For this review, take the finished solid that the model builds, in its own axes (mm). Face numbers are marked on the shaded views. Coordinates: 2 decimals unless noted, no trailing zeros. Loops run counter-clockwise (first coordinate to the right, second up) from the corner with the lowest first, then second, coordinate; pieces in that order, holes last. Notation, with made-up numbers: M 68.5,-33 L 100.5,-33 A26 cw 100.5,3 Z; hole C -7.75,46 d1. An arc over 180 degrees is marked long. Answer as a JSON object with one key per item and string values. Group by question number.
Item 1: Add section C-C (z = -20). State the section outline as (x, y) points.
Item 2: Add section D-D (x = 64.5). State the section outline as (y, z) points.
Item 3: Insertion check: pin 1 (1 mm diameter, centred on x = 36, z = -32.5, fed in from -Y). The pin has a flat end and moves straight along its axis. Give the tip position at first contact, or say it passes through.
Item 4: Add section A-A (y = -3.95). State the section outline as (x, z) points, then the cut area to 3 significant figures.
Item 5: Mouldability with a two-part tool opening along X and no side actions: class the marked faces 1 and 2 as +X half, -X half, draft (parallel to the pull), parting line (faces both ways), or undercut.
Item 6: Add section B-B (x = 26). State the section outline as (y, z) points.
Item 7: Wall thickness on L1, parallel to Z at x = 60.5, y = -2.7; L2, parallel to X at y = -3.3, z = -19; L3, parallel to X at y = -3.65, z = -7.5: over which ranges is each line inside the solid? List them lowest first. Write a range as from..to.
from build123d import *

# Parameters (mm, degrees)
F0_W     = 76.2
F0_H     = 38.1
F1_DEPTH = 5.08
F2_W     = 72.268962
F2_H     = 32.798988
F3_DEPTH = 2.54
F4_R     = 10.16
F5_DEPTH = 2.54


with BuildPart() as f1:
    # F0 (on Front) → F1 (new body)
    with BuildSketch(Plane.XZ):
        with Locations((38.1, -19.05)):
            Rectangle(F0_W, F0_H)
    extrude(amount=F1_DEPTH)

    # F2 (on face) → F3 (cut)
    with BuildSketch(Plane.XZ.offset(5.08)):
        with Locations((37.983545, -18.917193)):
            Rectangle(F2_W, F2_H)
    extrude(amount=-F3_DEPTH, mode=Mode.SUBTRACT)

    # F4 (on face) → F5 (join)
    with BuildSketch(Plane.XZ.offset(2.54)):
        with Locations((13.917368, -18.489809)):
            Circle(F4_R)
        with Locations((36.991507, -18.844597)):
            Circle(F4_R)
        with Locations((60.718681, -18.846158)):
            Circle(F4_R)
    extrude(amount=F5_DEPTH)


solid = f1.part
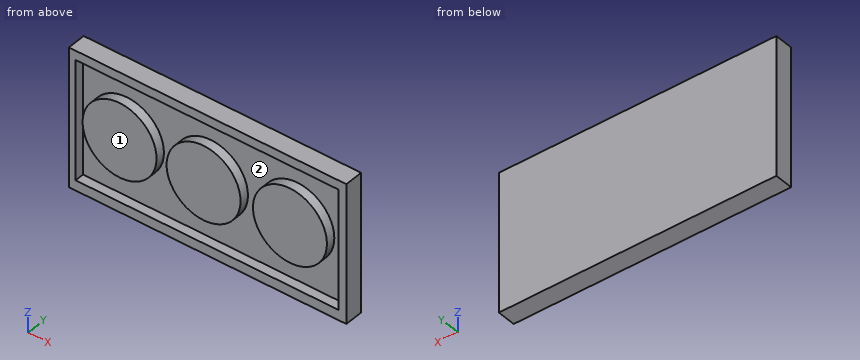
From the geometry:
{
 "1": {"outline": "M 0,-5.08 L 1.85,-5.08 L 1.85,-2.54 L 3.87,-2.54 L 3.87,-5.08 L 23.96,-5.08 L 23.96,-2.54 L 26.9,-2.54 L 26.9,-5.08 L 47.09,-5.08 L 47.09,-2.54 L 50.62,-2.54 L 50.62,-5.08 L 70.81,-5.08 L 70.81,-2.54 L 74.12,-2.54 L 74.12,-5.08 L 76.2,-5.08 L 76.2,0 L 0,0 Z"},
 "2": {"outline": "M -5.08,-38.1 L 0,-38.1 L 0,0 L -5.08,0 L -5.08,-2.52 L -2.54,-2.52 L -2.54,-9.42 L -5.08,-9.42 L -5.08,-28.28 L -2.54,-28.28 L -2.54,-35.32 L -5.08,-35.32 Z"},
 "3": {"pin 1": "stops at y = -2.54"},
 "4": {"outline": "M 0,-38.1 L 76.2,-38.1 L 76.2,0 L 0,0 Z; C 13.92,-18.49 d20.32; C 36.99,-18.84 d20.32; C 60.72,-18.85 d20.32; hole M 1.85,-35.32 L 74.12,-35.32 L 74.12,-2.52 L 1.85,-2.52 Z", "area": "1,510 mm²"},
 "5": {"face 1": "draft", "face 2": "undercut"},
 "6": {"outline": "M -5.08,-38.1 L 0,-38.1 L 0,0 L -5.08,0 L -5.08,-2.52 L -2.54,-2.52 L -2.54,-35.32 L -5.08,-35.32 Z"},
 "7": {"L1": "z = -38.1..-35.32, -29..-8.69, -2.52..0", "L2": "x = 0..1.85, 3.77..24.06, 26.83..47.15, 50.56..70.88, 74.12..76.2", "L3": "x = 0..1.85, 74.12..76.2"}
}
